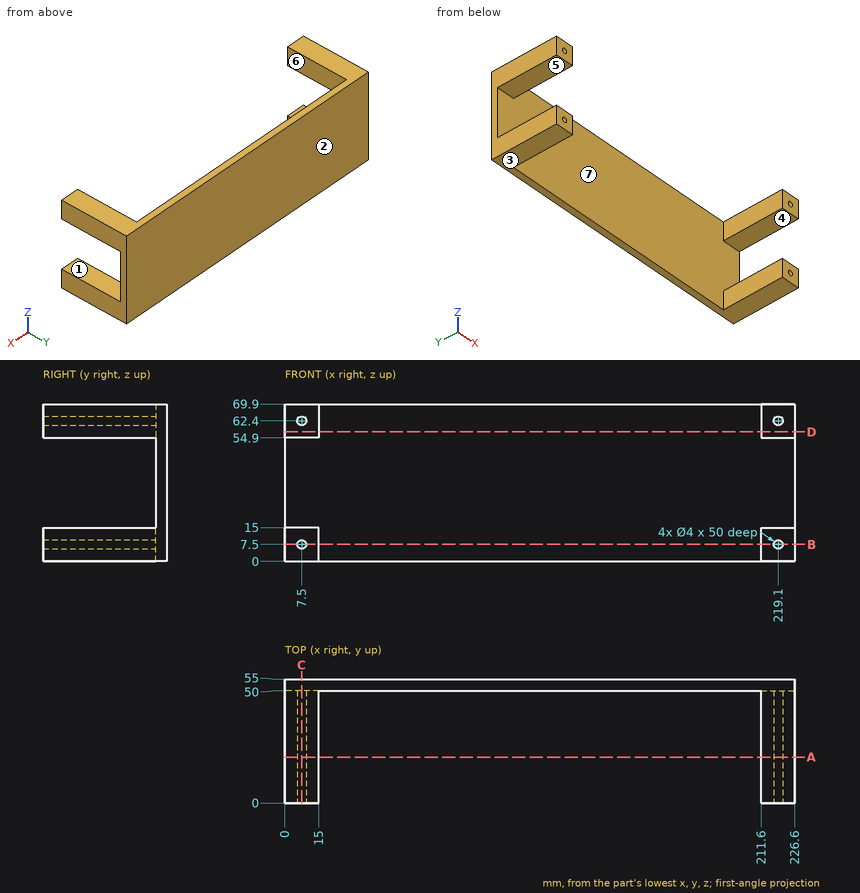
Check sheet for the drawn part. Datum: minimum x, y, z corner. Units: mm. A direction names the side the tool comes from. Coordinates: 2 decimals unless noted, no trailing zeros. Order: outer loops, then holes, each group sorted by start corner. A loop starts at its lowest first (then second) coordinate and runs counter-clockwise, first axis right, second up. Notation, with made-up numbers: M 66.25,19.5 L 91.25,19.5 A15 ccw 91.25,36.5 Z; hole C 26.25,78 d4. An arc over 180 degrees is marked long. One line per item, written item: value. Start each with the question number.
Item 1: Sectioned sample at B-B (z = 7.5). Enter the section's corners in (x, y), then the cut area to 3 significant figures.
Item 2: Gauge pin test, flat end, axial feed: pin 1 (2 mm diameter, centred on x = 219.5, z = 7, fed in from -Y). Record the tip position at first contact, or that the pin passes through.
Item 3: Sectioned sample at A-A (y = 20.5). Enter the section's corners in (x, z), then the cut area to 3 significant figures.
Item 4: Sectioned sample at C-C (x = 7.5). Enter the section's corners in (y, z), then the cut area to 3 significant figures.
Item 5: Scan lines: probe 1 along X at (y, z) = (19, 7.5); probe 2 along Z at (x, y) = (219, 12); probe 3 along X at (y, z) = (14, 7). Record each from-to range of solid material in increasing order.
Item 6: Sectioned sample at D-D (z = 57.5). Enter the section's corners in (x, y), then the cut area to 3 significant figures.
Item 7: Access from +Z, -Z, +X, -X, +Y, -Y to the whole of each face (thin tool, end or side, straight path). Record for the marked faces 5, 6 and 7.
Item 8: Mould release check, pull along Z, two halves, no side actions. Record for the marked faces 1, 2, 3 and 4: released by +Z, released by -Z, zero draft, split by the parting line, or undercut.
Conclusion:
1. outline: M 0,0 L 5.5,0 L 5.5,50 L 9.5,50 L 9.5,0 L 15,0 L 15,50 L 211.6,50 L 211.6,0 L 217.1,0 L 217.1,50 L 221.1,50 L 221.1,0 L 226.6,0 L 226.6,55 L 0,55 Z
1. area: 2,230 mm^2
2. pin 1: stops at y = 50
3. outline: M 0,0 L 15,0 L 15,15 L 0,15 Z; M 0,54.9 L 15,54.9 L 15,69.9 L 0,69.9 Z; M 211.6,0 L 226.6,0 L 226.6,15 L 211.6,15 Z; M 211.6,54.9 L 226.6,54.9 L 226.6,69.9 L 211.6,69.9 Z; hole C 7.5,7.5 d4; hole C 7.5,62.4 d4; hole C 219.1,7.5 d4; hole C 219.1,62.4 d4
3. area: 850 mm^2
4. outline: M 0,0 L 55,0 L 55,69.9 L 0,69.9 L 0,64.4 L 50,64.4 L 50,60.4 L 0,60.4 L 0,54.9 L 50,54.9 L 50,15 L 0,15 L 0,9.5 L 50,9.5 L 50,5.5 L 0,5.5 Z
4. area: 1,450 mm^2
5. probe 1: x = 0 to 5.5, 9.5 to 15, 211.6 to 217.1, 221.1 to 226.6
5. probe 2: z = 0 to 5.5, 9.5 to 15, 54.9 to 60.4, 64.4 to 69.9
5. probe 3: x = 0 to 5.56, 9.44 to 15, 211.6 to 217.16, 221.04 to 226.6
6. outline: M 0,0 L 15,0 L 15,50 L 211.6,50 L 211.6,0 L 226.6,0 L 226.6,55 L 0,55 Z
6. area: 2,630 mm^2
7. face 5: +X, -X, -Y
7. face 6: +Z, -Z, -Y
7. face 7: -Y
8. face 1: undercut
8. face 2: zero draft
8. face 3: released by -Z
8. face 4: undercut
